```python
from build123d import *

# Parameters (mm, degrees)
SKETCH1_W           = 133
SKETCH1_H           = 44
BOSS_EXTRUDE1_DEPTH = 20
BOSS_EXTRUDE3_DEPTH = 20


with BuildPart() as part:
    # Sketch1 → Boss-Extrude1 (new body)
    with BuildSketch(Plane(origin=(0, 0, 0), x_dir=(1, 0, 0), z_dir=(0, 1, 0))):
        Rectangle(SKETCH1_W, SKETCH1_H)
    extrude(amount=BOSS_EXTRUDE1_DEPTH)

    # Sketch2 → Boss-Extrude3 (add)
    with BuildSketch(Plane.ZY.offset(66.5)):
        with BuildLine():
            ThreePointArc((-18, 12.25), (-18.775155536, 13.831061681), (-20.499756038, 14.186554647))
            Line((-20.499756038, 14.186554647), (-20, 12.25))
            Line((-20, 12.25), (-20, 10.25))
            ThreePointArc((-20, 10.25), (-18.585786438, 10.835786438), (-18, 12.25))
        make_face()
        with BuildLine():
            Line((-20, 12.25), (-20.499756038, 14.186554647))
            ThreePointArc((-20.499756038, 14.186554647), (-21.984075263, 11.998116391), (-20, 10.25))
            Line((-20, 10.25), (-20, 12.25))
        make_face()
        with BuildLine():
            ThreePointArc((-18, 7.75), (-18.585786438, 9.164213562), (-20, 9.75))
            Line((-20, 9.75), (-20, 7.75))
            Line((-20, 7.75), (-20.499756038, 5.813445353))
            ThreePointArc((-20.499756038, 5.813445353), (-18.775155536, 6.168938319), (-18, 7.75))
        make_face()
        with BuildLine():
            Line((-20, 7.75), (-20, 9.75))
            ThreePointArc((-20, 9.75), (-21.984075263, 8.001883609), (-20.499756038, 5.813445353))
            Line((-20.499756038, 5.813445353), (-20, 7.75))
        make_face()
        with BuildLine():
            ThreePointArc((22, 15.25), (21.709864781, 16.136694542), (20.951697052, 16.680373998))
            Line((20.951697052, 16.680373998), (20.5, 15.25))
            Line((20.5, 15.25), (20.5, 13.75))
            ThreePointArc((20.5, 13.75), (21.560660172, 14.189339828), (22, 15.25))
        make_face()
        with BuildLine():
            Line((20.5, 15.25), (20.951697052, 16.680373998))
            ThreePointArc((20.951697052, 16.680373998), (19.017508685, 15.478515868), (20.5, 13.75))
            Line((20.5, 13.75), (20.5, 15.25))
        make_face()
        with BuildLine():
            ThreePointArc((22, 11.75), (21.560660172, 12.810660172), (20.5, 13.25))
            Line((20.5, 13.25), (20.5, 11.75))
            Line((20.5, 11.75), (20.5, 10.25))
            ThreePointArc((20.5, 10.25), (21.560660172, 10.689339828), (22, 11.75))
        make_face()
        with BuildLine():
            Line((20.5, 11.75), (20.5, 13.25))
            ThreePointArc((20.5, 13.25), (19, 11.75), (20.5, 10.25))
            Line((20.5, 10.25), (20.5, 11.75))
        make_face()
        with BuildLine():
            ThreePointArc((22, 8.25), (21.560660172, 9.310660172), (20.5, 9.75))
            Line((20.5, 9.75), (20.5, 8.25))
            Line((20.5, 8.25), (20.5, 6.75))
            ThreePointArc((20.5, 6.75), (21.560660172, 7.189339828), (22, 8.25))
        make_face()
        with BuildLine():
            Line((20.5, 8.25), (20.5, 9.75))
            ThreePointArc((20.5, 9.75), (19, 8.25), (20.5, 6.75))
            Line((20.5, 6.75), (20.5, 8.25))
        make_face()
        with BuildLine():
            ThreePointArc((22, 4.75), (21.560660172, 5.810660172), (20.5, 6.25))
            Line((20.5, 6.25), (20.5, 4.75))
            Line((20.5, 4.75), (20.951697052, 3.319626002))
            ThreePointArc((20.951697052, 3.319626002), (21.709864781, 3.863305458), (22, 4.75))
        make_face()
        with BuildLine():
            Line((20.5, 4.75), (20.5, 6.25))
            ThreePointArc((20.5, 6.25), (19.017508685, 4.521484132), (20.951697052, 3.319626002))
            Line((20.951697052, 3.319626002), (20.5, 4.75))
        make_face()
    extrude(amount=BOSS_EXTRUDE3_DEPTH)


solid = part.part
```
Geometry: final body of the model. Coordinates: model frame, mm. Round coordinates to 2 decimals unless told otherwise and drop trailing zeros. Write each loop counter-clockwise with the first axis right and the second up, starting at its lowest first coordinate (ties: lowest second). Pieces come first, ordered by that corner, then holes. Notation, with made-up numbers: M 78.5,-13 L 100.5,-13 A25 ccw 100.5,3 Z; hole C -34,81.5 d4. An arc over 180 degrees is marked long. Answer in a Markdown table with one row per item. Add a question column.
(1) Contact query for a flat-ended pin moving along its axis: pin 1 (4 mm diameter, centred on x = -69.5, y = 3.5, fed in from +Z). Output: stop coordinate, or through.
(2) Draft query along Z for faces 1 (the face through (-66.5, 10, 0)), 2 (the face through (-1, 10, 22)), 3 (the face through (-1, 0, 0)). Return one class per face: pulls with the +Z half, pulls with the -Z half, needs draft (parallel to the pull), parting line crosses it, or undercut.
(3) Cut plane A-A, the plane z = -10.5. Return the cut outline in (x, y), then the cut area to 3 significant figures.
(4) Ray query, L1, parallel to X at y = 2.5, z = 11; L2, parallel to Z at x = -80, y = 11.5. Return the intervals inside material, ascending.
Established:
| question | item | result |
|---|---|---|
| 1 | pin 1 | z = 22 |
| 2 | face 1 | undercut |
| 2 | face 2 | pulls with the +Z half |
| 2 | face 3 | needs draft |
| 3 | outline | M -66.5,0 L 66.5,0 L 66.5,20 L -66.5,20 Z |
| 3 | area | 2,660 mm² |
| 4 | L1 | -66.5 to 66.5 |
| 4 | L2 | -21.85 to -18.15, 19.02 to 21.98 |
